Check sheet for the modelled part. Datum: model origin and axes. Units: mm. A direction names the side the tool comes from. Round coordinates to 2 decimals unless told otherwise and drop trailing zeros. Order: outer loops, then holes, each group sorted by start corner. A loop starts at its lowest first (then second) coordinate and runs counter-clockwise, first axis right, second up. Notation, with made-up numbers: (-20.5, 45.25) -> (10.5, 45.25) arc R27 ccw to (10.5, 79.25) -> close; hole circle Ø9 at (-37, -23). An arc over 180 degrees is marked (long way). Answer in a Markdown table with one row per item.
from build123d import *

# Parameters (mm, degrees)
RESSALTO_EXTRUS_O1_DEPTH = 4
ESBO_O2_OUTSIDE_W        = 124.534
ESBO_O2_OUTSIDE_H        = 125.772
ESBO_O2_OUTSIDE_R        = 3.5
CORTE_EXTRUS_O1_DEPTH    = 15
CORTE_EXTRUS_O1_DRAFT    = -75
ESBO_O3_OUTSIDE_W        = 124.534
ESBO_O3_OUTSIDE_H        = 125.772
ESBO_O3_OUTSIDE_R        = 3.5
CORTE_EXTRUS_O5_DEPTH    = 15
CORTE_EXTRUS_O5_DRAFT    = -75
ESBO_O9_R                = 3
RESSALTO_EXTRUS_O2_DEPTH = 14


with BuildPart() as part:
    # Esboço1 → Ressalto-extrusão1 (new body)
    with BuildSketch(Plane.XY):
        Polygon((0, -4.618802154), (4, -2.309401077), (4, 2.309401077), (0, 4.618802154), (-4, 2.309401077), (-4, -2.309401077), align=None)
    extrude(amount=RESSALTO_EXTRUS_O1_DEPTH)


with BuildPart() as corte_extrus_o1_tool:
    # Esboço2 outside → Corte-extrusão1 (with draft: the straight prism first)
    with BuildSketch(Plane.XY.offset(4)):
        Rectangle(ESBO_O2_OUTSIDE_W, ESBO_O2_OUTSIDE_H)
        Circle(ESBO_O2_OUTSIDE_R, mode=Mode.SUBTRACT)
    extrude(amount=-CORTE_EXTRUS_O1_DEPTH)
    # Corte-extrusão1: the draft: its side faces are tilted about the plane it starts from
    corte_extrus_o1_sides = [corte_extrus_o1_tool.faces().sort_by_distance(p)[0] for p in [
        (0, -62.886, -3.5),
        (62.267, 0, -3.5),
        (0, 62.886, -3.5),
        (-62.267, 0, -3.5),
        (-3.5, 0, -3.5),
    ]]
    draft(corte_extrus_o1_sides, Plane.XY.offset(4), CORTE_EXTRUS_O1_DRAFT)


with BuildPart() as part_1:
    add(part.part)

    # Corte-extrusão1: cut by corte_extrus_o1_tool
    add(corte_extrus_o1_tool.part, mode=Mode.SUBTRACT)


with BuildPart() as corte_extrus_o5_tool:
    # Esboço3 outside → Corte-extrusão5 (with draft: the straight prism first)
    with BuildSketch(Plane(origin=(0, 0, 0), x_dir=(-1, 0, 0), z_dir=(0, 0, -1))):
        Rectangle(ESBO_O3_OUTSIDE_W, ESBO_O3_OUTSIDE_H)
        Circle(ESBO_O3_OUTSIDE_R, mode=Mode.SUBTRACT)
    extrude(amount=-CORTE_EXTRUS_O5_DEPTH)
    # Corte-extrusão5: the draft: its side faces are tilted about the plane it starts from
    corte_extrus_o5_sides = [corte_extrus_o5_tool.faces().sort_by_distance(p)[0] for p in [
        (0, -62.886, 7.5),
        (-62.267, 0, 7.5),
        (0, 62.886, 7.5),
        (62.267, 0, 7.5),
        (3.5, 0, 7.5),
    ]]
    draft(corte_extrus_o5_sides, Plane(origin=(0, 0, 0), x_dir=(-1, 0, 0), z_dir=(0, 0, -1)), CORTE_EXTRUS_O5_DRAFT)


with BuildPart() as part_2:
    add(part_1.part)

    # Corte-extrusão5: cut by corte_extrus_o5_tool
    add(corte_extrus_o5_tool.part, mode=Mode.SUBTRACT)

    # Esboço9 → Ressalto-extrusão2 (add)
    with BuildSketch(Plane(origin=(0, 0, 0), x_dir=(-1, 0, 0), z_dir=(0, 0, -1))):
        Circle(ESBO_O9_R)
    extrude(amount=RESSALTO_EXTRUS_O2_DEPTH)


solid = part_2.part
Item 1: Depth check by flat-ended pin: P1, Ø3, axis at x = 1, z = -12, coming from the +Y side; P2, Ø1.5, axis at x = -2, z = -3.5, coming from the +Y side. Enter the tip coordinate at first touch or a pass-through.
Result sheet:
| item | result |
|---|---|
| P1 | stops at y = 3 |
| P2 | stops at y = 2.73 |
Item 2: Set-up check for faces 1 (the flat face through (3, 1, 0)), 2 (the flat face through (-2.028, -3.448, 1.974)): record each of +Z, -Z, +X, -X, +Y, -Y from which the full face is reachable in a straight line by a thin tool's end or side.
Result sheet:
| item | result |
|---|---|
| face 1 | -Z |
| face 2 | +Z, -Z, -X, -Y |
Item 3: Cross-section at B-B (z = -3.75). Record the boundary of the cut face in (x, y).
Result sheet:
| item | result |
|---|---|
| outline | circle Ø6 at (0, 0) |
Item 4: Cross-section at A-A (y = 0). Record the boundary of the cut face in (x, z), and give its area (3 significant figures).
Result sheet:
| item | result |
|---|---|
| outline | (-4, 0.13) -> (-3.5, 0) -> (-3, 0) -> (-3, -14) -> (3, -14) -> (3, 0) -> (3.5, 0) -> (4, 0.13) -> (4, 3.87) -> (3.5, 4) -> (-3.5, 4) -> (-4, 3.87) -> close |
| area | 116 mm^2 |
Item 5: Cross-section at C-C (z = 2.75). Record the boundary of the cut face in (x, y), and give its area (3 significant figures).
Result sheet:
| item | result |
|---|---|
| outline | (-4, -2.31) -> (0, -4.62) -> (4, -2.31) -> (4, 2.31) -> (0, 4.62) -> (-4, 2.31) -> close |
| area | 55.4 mm^2 |
Item 6: Scan lines: line 1 (Z direction, x = -1.5, y = 3); line 2 (Y direction, x = 0, z = -10.25); line 3 (X direction, y = 4, z = 0.25). Record each from-to range of solid material in increasing order. Write a range as [from, to].
Result sheet:
| item | result |
|---|---|
| line 1 | z = [0, 4] |
| line 2 | y = [-3, 3] |
| line 3 | x = [-1.07, 1.07] |
